```python
from build123d import *

# Parameters (mm, degrees)
ESBO_O1_W                = 10
ESBO_O1_H                = 6
RESSALTO_EXTRUS_O1_DEPTH = 3


with BuildPart() as part:
    # Esboço1 → Ressalto-extrusão1 (new body)
    with BuildSketch(Plane.XY):
        Polygon((-12.5, 16), (-12.5, -16), (-5, -16), (5, -16), (12.5, -16), (12.5, -7.5), (-2.5, -7.5), (-2.5, 7.5), (12.5, 7.5), (12.5, 16), (5, 16), (-5, 16), align=None)
        with Locations((0, 19)):
            Rectangle(ESBO_O1_W, ESBO_O1_H)
        with Locations((0, -19)):
            Rectangle(ESBO_O1_W, ESBO_O1_H)
    extrude(amount=RESSALTO_EXTRUS_O1_DEPTH)


solid = part.part
```
Build history of the part. All positions in model axes, mm. A direction names the side the tool comes from. Round coordinates to 2 decimals unless told otherwise and drop trailing zeros. Loops run counter-clockwise (first coordinate to the right, second up) from the corner with the lowest first, then second, coordinate; pieces in that order, holes last.
Item 1: Two-plate mould, pull along Y, no slides. Class faces 5 (the face through (5, 7.5, 1)), 6 (the face through (12.5, 12, 1)), 7 (the face through (-9, 16, 1)): released by +Y, released by -Y, zero draft, split by the parting line, or undercut.
Item 2: Pin check, flat tips, straight feed: P1, Ø8, axis at x = -2.5, y = -3.5, coming from the -Z side; P2, Ø1.5, axis at y = 18.5, z = 2, coming from the +X side; P3, Ø1.5, axis at x = 6.5, z = 0.5, coming from the +Y side. Stop position of each tip, or through.
Item 3: Saw through at D-D (x = -7.5). List the corners of the cut face in (y, z), then the cut area to 3 significant figures.
Item 4: Saw through at A-A (x = 2.5). List the corners of the cut face in (y, z).
Item 5: Saw through at C-C (y = -3). List the corners of the cut face in (x, z).
Item 6: Saw through at B-B (z = 0.9). List the corners of the cut face in (x, y), then the cut area to 3 significant figures.
Item 7: Drill centre lines: line 1 along Y through (x, z) = (11.75, 0.3); line 2 along Y through (x, z) = (1.25, 2); line 3 along X through (y, z) = (19, 0.55). Where is each one in solid material? Low to high.
Item 8: Which spindle directions (+Z, -Z, +X, -X, +Y, -Y) get a long thin tool onto all of the face, cutting with end or side? Do faces 1 (the face through (-5, -19, 1)), 2 (the face through (-5, 19, 1)), 3 (the face through (9, -16, 1)), 4 (the face through (9, 16, 1)). Say none if no direction does.
Worked answers:
1. face 5: undercut
1. face 6: zero draft
1. face 7: released by +Y
2. P1: stops at z = 0
2. P2: stops at x = 5
2. P3: stops at y = 16
3. outline: (-16, 0) - (16, 0) - (16, 3) - (-16, 3) - close
3. area: 96.0 mm2
4. outline: (-22, 0) - (-7.5, 0) - (-7.5, 3) - (-22, 3) - close; (7.5, 0) - (22, 0) - (22, 3) - (7.5, 3) - close
5. outline: (-12.5, 0) - (-2.5, 0) - (-2.5, 3) - (-12.5, 3) - close
6. outline: (-12.5, -16) - (-5, -16) - (-5, -22) - (5, -22) - (5, -16) - (12.5, -16) - (12.5, -7.5) - (-2.5, -7.5) - (-2.5, 7.5) - (12.5, 7.5) - (12.5, 16) - (5, 16) - (5, 22) - (-5, 22) - (-5, 16) - (-12.5, 16) - close
6. area: 695 mm2
7. line 1: y = -16 to -7.5, 7.5 to 16
7. line 2: y = -22 to -7.5, 7.5 to 22
7. line 3: x = -5 to 5
8. face 1: +Z, -Z, -X, -Y
8. face 2: +Z, -Z, -X, +Y
8. face 3: +Z, -Z, +X, -Y
8. face 4: +Z, -Z, +X, +Y
